from build123d import *

# Parameters (mm, degrees)
SCHIZZO1_W                     = 30
SCHIZZO1_H                     = 30
SCHIZZO1_R                     = 6
ESTRUSIONE_ESTRUSIONE1_DEPTH   = 30
F_8_0_8_DIAMETER_HOLE1_D       = 8
F_8_0_8_DIAMETER_HOLE1_DEPTH   = 12
F_8_0_8_DIAMETER_HOLE1_TIP     = 2.403442476
FORO_FILETTATO_M3_1_AT_2_COUNT = 2
FORO_FILETTATO_M3_1_AT_2_PITCH = 20
SKETCH1_R                      = 1.25
CUT_EXTRUDE1_DEPTH             = 10


with BuildPart() as part:
    # Schizzo1 → Estrusione-Estrusione1 (new body)
    with BuildSketch(Plane.XY):
        with Locations((15, 15)):
            Rectangle(SCHIZZO1_W, SCHIZZO1_H)
        with Locations((12, 16.8)):
            Circle(SCHIZZO1_R, mode=Mode.SUBTRACT)
    extrude(amount=ESTRUSIONE_ESTRUSIONE1_DEPTH)

    # Ø8.0 (8) Diameter Hole1
    with Locations(Plane(origin=(30, 0, 0), x_dir=(0, 0, -1), z_dir=(1, 0, 0))):
        with Locations((-15, 10)):
            Hole(F_8_0_8_DIAMETER_HOLE1_D / 2, depth=F_8_0_8_DIAMETER_HOLE1_DEPTH)
            with Locations((0, 0, -(F_8_0_8_DIAMETER_HOLE1_DEPTH + F_8_0_8_DIAMETER_HOLE1_TIP / 2))):  # 118° drill point
                Cone(0, F_8_0_8_DIAMETER_HOLE1_D / 2, F_8_0_8_DIAMETER_HOLE1_TIP, mode=Mode.SUBTRACT)

    # Schizzo7 → Foro filettato M3-1 (revolve, cut)
    with BuildSketch(Plane(origin=(5, 30, 25), x_dir=(0, 0, 1), z_dir=(1, 0, 0))):
        Polygon((0, 0), (0, 9.251075774), (1.25, 8.5), (1.25, 0.158771324), (1.525, 0), align=None)
    foro_filettato_m3_1 = revolve(axis=Axis((5, 36.35, 25), (0, -1, 0)), mode=Mode.SUBTRACT)

    # Foro filettato M3-1 at 2: Foro filettato M3-1 ×2
    with Locations(*[(i * FORO_FILETTATO_M3_1_AT_2_PITCH, 0, 0) for i in range(1, FORO_FILETTATO_M3_1_AT_2_COUNT)]):
        add(foro_filettato_m3_1, mode=Mode.SUBTRACT)

    # Specchia1: Foro filettato M3-1 across plane
    add(foro_filettato_m3_1.mirror(Plane.XY.offset(15)), mode=Mode.SUBTRACT)

    # Specchia1 copy 1 sketch → Specchia1 copy 1 (revolve, cut)
    with BuildSketch(Plane(origin=(25, 30, 5), x_dir=(0, 0, -1), z_dir=(1, 0, 0))):
        Polygon((0, 0), (0, -9.251075774), (1.25, -8.5), (1.25, -0.158771324), (1.525, 0), align=None)
    revolve(axis=Axis((25, 36.35, 5), (0, 1, 0)), mode=Mode.SUBTRACT)

    # Sketch1 → Cut-Extrude1 (cut)
    with BuildSketch(Plane.XZ):
        with Locations(Location((25, 15, 0), (0, 0, 270))):
            Circle(SKETCH1_R)
    extrude(amount=-CUT_EXTRUDE1_DEPTH, mode=Mode.SUBTRACT)


solid = part.part
Geometry: final body of the model. Coordinates: model frame, mm. A direction names the side the tool comes from. Round coordinates to 2 decimals unless told otherwise and drop trailing zeros. Order: outer loops, then holes, each group sorted by start corner. A loop starts at its lowest first (then second) coordinate and runs counter-clockwise, first axis right, second up.
Q1. Section D-D, the plane x = 28. Output: boundary loops of the cut face in (y, z).
Result sheet:
outline: (0, 0) - (30, 0) - (30, 30) - (0, 30) - close; hole circle Ø8 at (10, 15)
Q2. Section C-C, the plane z = 7.5. Output: boundary loops of the cut face in (x, y), and give its area (3 significant figures).
Result sheet:
outline: (0, 0) - (30, 0) - (30, 30) - (0, 30) - close; hole circle Ø12 at (12, 16.8)
area: 787 mm2
Q3. Mould query, pull axis X, two halves, no side actions, for faces 1 (the face through (16.014, 10.586, 14.627)), 2 (the face through (0, 15, 15)), 3 (the face through (25.05, 3.06, 16.25)). Classes: released by +X, released by -X, zero draft, split by the parting line, or undercut.
Result sheet:
face 1: released by +X
face 2: released by -X
face 3: undercut
Q4. Section A-A, the plane y = 16.8. Output: boundary loops of the cut face in (x, z), and give its area (3 significant figures).
Result sheet:
outline: (0, 0) - (6, 0) - (6, 30) - (0, 30) - close; (18, 0) - (30, 0) - (30, 30) - (18, 30) - close
area: 540 mm2
Q5. Pin query (flat end, axial travel): pin 1 (4 mm diameter, centred on x = 25.5, z = 15.5, fed in from -Y); pin 2 (2 mm diameter, centred on x = 5, z = 5, fed in from +Y); pin 3 (6.5 mm diameter, centred on y = 10, z = 15, fed in from +X); pin 4 (3 mm diameter, centred on x = 25, z = 25, fed in from +Y). Return the tip coordinate at first contact, or that it passes through.
Result sheet:
pin 1: stops at y = 0
pin 2: stops at y = 21.35
pin 3: stops at x = 17.55
pin 4: stops at y = 29.99
Q6. Material intervals for probe 1 along X at (y, z) = (25.25, 5); probe 2 along X at (y, z) = (4, 15), sorted ascending.
Result sheet:
probe 1: x = 0 to 3.75, 6.25 to 23.75, 26.25 to 30
probe 2: x = 0 to 23.75, 26.25 to 30
Q7. Section B-B, the plane x = 12. Output: boundary loops of the cut face in (y, z), and give its area (3 significant figures).
Result sheet:
outline: (0, 0) - (10.8, 0) - (10.8, 30) - (0, 30) - close; (22.8, 0) - (30, 0) - (30, 30) - (22.8, 30) - close
area: 540 mm2
Q8. Access query for faces 4 (the face through (23.916, 13.966, 14.479)), 5 (the face through (30, 15, 15)), 6 (the face through (25.479, 25.729, 26.155)). Directions: +Z, -Z, +X, -X, +Y, -Y. A direction counts if a zero-diameter tool reaches every point of the face in a straight line with its end or side. Return the directions, or none.
Result sheet:
face 4: +X
face 5: +Z, -Z, +X, +Y, -Y
face 6: +Y
